```python
from build123d import *

# Parameters (mm, degrees)
SKETCH1_R           = 1.7
BOSS_EXTRUDE1_DEPTH = 11.7
SKETCH2_R           = 2.25
CUT_EXTRUDE1_DEPTH  = 101.718518655
BOSS_EXTRUDE2_START = -2
SKETCH3_R           = 1.5
BOSS_EXTRUDE2_DEPTH = 3
BOSS_EXTRUDE3_START = -19
SKETCH3_2_R         = 1.5
BOSS_EXTRUDE3_DEPTH = 3


with BuildPart() as part:
    # Sketch1 → Boss-Extrude1 (new, symmetric)
    with BuildSketch(Plane(origin=(0, 0, 0), x_dir=(1, 0, 0), z_dir=(0, 1, 0))):
        with BuildLine():
            Line((60, 94.2), (65.5, 99.7))
            Line((65.5, 99.7), (65.5, 55.681623382))
            Line((65.5, 55.681623382), (61.909188309, 52.090811691))
            ThreePointArc((61.909188309, 52.090811691), (57.505525262, 52.966754733), (60, 56.7))
            Line((60, 56.7), (60, 82.3))
            ThreePointArc((60, 82.3), (62.7, 85), (60, 87.7))
            Line((60, 87.7), (60, 88.7))
            Line((60, 88.7), (60, 93.2))
            Line((60, 93.2), (60, 94.2))
        make_face()
        with Locations(Location((60, 54, 0), (0, 0, 270))):
            Circle(SKETCH1_R, mode=Mode.SUBTRACT)
    extrude(amount=BOSS_EXTRUDE1_DEPTH, both=True)

    # Sketch2 → Cut-Extrude1 (cut, through all)
    with BuildSketch(Plane(origin=(65.5, 0, 0), x_dir=(0, 0, -1), z_dir=(1, 0, 0))):
        with Locations((90.95, 1.45)):
            Circle(SKETCH2_R)
    extrude(amount=-CUT_EXTRUDE1_DEPTH, mode=Mode.SUBTRACT)

    # Sketch3 → Boss-Extrude2 (add)
    with BuildSketch(Plane.XZ.offset(11.7).offset(BOSS_EXTRUDE2_START)):
        with BuildLine():
            Line((52.5, -66.8), (60, -66.8))
            Line((60, -66.8), (60, -72.2))
            Line((60, -72.2), (52.5, -72.2))
            ThreePointArc((52.5, -72.2), (49.8, -69.5), (52.5, -66.8))
        make_face()
        with Locations(Location((52.5, -69.5, 0), (0, 0, 270))):
            Circle(SKETCH3_R, mode=Mode.SUBTRACT)
    extrude(amount=-BOSS_EXTRUDE2_DEPTH)

    # Sketch3_2 → Boss-Extrude3 (add)
    with BuildSketch(Plane.XZ.offset(11.7).offset(BOSS_EXTRUDE3_START)):
        with BuildLine():
            Line((52.5, -66.8), (60, -66.8))
            Line((60, -66.8), (60, -72.2))
            Line((60, -72.2), (52.5, -72.2))
            ThreePointArc((52.5, -72.2), (49.8, -69.5), (52.5, -66.8))
        make_face()
        with Locations(Location((52.5, -69.5, 0), (0, 0, 270))):
            Circle(SKETCH3_2_R, mode=Mode.SUBTRACT)
    extrude(amount=-BOSS_EXTRUDE3_DEPTH)


solid = part.part
```
Source: CAD feature listing. Evaluate the final solid. Frame: model axes, mm. A direction names the side the tool comes from. Coordinates: 2 decimals unless noted, no trailing zeros. Loops run counter-clockwise (first coordinate to the right, second up) from the corner with the lowest first, then second, coordinate; pieces in that order, holes last. Notation, with made-up numbers: (68.25, 35.5) -> (126.25, 35.5) arc R30 cw to (126.25, 64.5) -> close; hole circle Ø4 at (54.25, 34.5). An arc over 180 degrees is marked (long way). One line per item, written item: value. Start each with the question number.
Q1. Set-up query: faces 4 (the face through (56, -9.7, -69)), 5 (the face through (56, 7.3, -69)), 6 (the face through (56, 9, -66.8)), 7 (the face through (56, -8, -72.2)), 8 (the face through (65.5, 0, -78)). Return all of +Z, -Z, +X, -X, +Y, -Y with unobstructed straight access to the full face (end or side cutting, diameter ignored); none if empty.
Q2. Section query A-A, the plane z = -69.5. Return the cut outline in (x, y), and give its area (3 significant figures).
Q3. Line query: line 1 along X through (y, z) = (7.9, -69.5); line 2 along Y through (x, z) = (61.55, -90.95); line 3 along X through (y, z) = (10, -91). Output: solid intervals per line, ascending.
Q4. Section query B-B, the plane y = 1.45. Return the cut outline in (x, z).
Q5. Mould query, pull axis X, two halves, no side actions, for faces 1 (the face through (49.8, 8.8, -69.6)), 2 (the face through (56, 9, -72.2)), 3 (the face through (51.925, -8.221, -70.886)). Classes: pulls with the +X half, pulls with the -X half, needs draft (parallel to the pull), parting line crosses it, or undercut.
Q6. Section query C-C, the plane x = 60.75. Return the cut outline in (y, z).
Q7. Section query D-D, the plane y = -1.25. Return the cut outline in (x, z), and give its area (3 significant figures).
Q8. Contact query for flat-ended pins moving along their axis: P1, Ø1.5, axis at x = 57, y = 8, coming from the -Z side; P2, Ø6, axis at x = 61.5, y = 3.5, coming from the -Z side; P3, Ø3.5, axis at y = 1.45, z = -90.95, coming from the +X side; P4, Ø6, axis at x = 54.5, z = -69, coming from the -Y side. Output: stop coordinate, or through.
Results:
1. face 4: -Z, -X, -Y
1. face 5: -Z, -X
1. face 6: -X, +Y, -Y
1. face 7: -Z, -X, +Y, -Y
1. face 8: +Z, -Z, +X, +Y, -Y
2. outline: (49.8, -9.7) -> (51, -9.7) -> (51, -6.7) -> (49.8, -6.7) -> close; (49.8, 7.3) -> (51, 7.3) -> (51, 10.3) -> (49.8, 10.3) -> close; (54, -9.7) -> (60, -9.7) -> (60, -11.7) -> (65.5, -11.7) -> (65.5, 11.7) -> (60, 11.7) -> (60, 10.3) -> (54, 10.3) -> (54, 7.3) -> (60, 7.3) -> (60, -6.7) -> (54, -6.7) -> close
2. area: 172 mm^2
3. line 1: 49.8 to 51, 54 to 65.5
3. line 2: -11.7 to -0.8, 3.7 to 11.7
3. line 3: 60 to 65.5
4. outline: (60, -94.2) -> (65.5, -99.7) -> (65.5, -93.2) -> (60, -93.2) -> close; (60, -88.7) -> (65.5, -88.7) -> (65.5, -55.68) -> (61.91, -52.09) arc R2.7 ccw (long way) to (60, -56.7) -> (60, -82.3) arc R2.7 cw to (60, -87.7) -> close; hole circle Ø3.4 at (60, -54)
5. face 1: pulls with the -X half
5. face 2: needs draft
5. face 3: undercut
6. outline: (-11.7, -94.95) -> (11.7, -94.95) -> (11.7, -87.59) -> (-11.7, -87.59) -> close; (-11.7, -82.41) -> (11.7, -82.41) -> (11.7, -55.53) -> (-11.7, -55.53) -> close; (-11.7, -52.47) -> (11.7, -52.47) -> (11.7, -51.41) -> (-11.7, -51.41) -> close; hole circle Ø4.5 at (1.45, -90.95)
7. outline: (60, -94.2) -> (65.5, -99.7) -> (65.5, -55.68) -> (61.91, -52.09) arc R2.7 ccw (long way) to (60, -56.7) -> (60, -82.3) arc R2.7 cw to (60, -87.7) -> close; hole circle Ø3.4 at (60, -54)
7. area: 232 mm^2
8. P1: z = -72.2
8. P2: z = -98.7
8. P3: through
8. P4: y = -9.7
